```python
from build123d import *

# Parameters (mm, degrees)
SKETCH_W        = 19
SKETCH_H        = 14
PAD_DEPTH       = 19
THICKNESS_T     = 3
SKETCH001_R     = 1.5
POCKET_DEPTH    = 20
SKETCH002_R     = 1.5
POCKET001_DEPTH = 3
CHAMFER_SIZE    = 1.5
SKETCH003_W     = 19
SKETCH003_H     = 25
PAD001_DEPTH    = 1
POCKET002_DEPTH = 24


with BuildPart() as part:
    # Sketch → Pad (new body)
    with BuildSketch(Plane.XY):
        Rectangle(SKETCH_W, SKETCH_H)
    extrude(amount=PAD_DEPTH)

    # Thickness
    thickness_openings = [part.faces().sort_by_distance(p)[0] for p in [
        (-9.5, 0, 9.5),
        (9.5, 0, 9.5),
    ]]
    offset(amount=THICKNESS_T, openings=thickness_openings, kind=Kind.INTERSECTION)

    # Sketch001 (on Face8 of Thickness) → Pocket (cut)
    with BuildSketch(Plane.XZ.offset(10)):
        with Locations((0, 9.5)):
            Circle(SKETCH001_R)
    extrude(amount=-POCKET_DEPTH, mode=Mode.SUBTRACT)

    # Sketch002 (on Face10 of Pocket) → Pocket001 (cut)
    with BuildSketch(Plane.XZ.offset(10)):
        with Locations((-6.25, 9.5)):
            Circle(SKETCH002_R)
        with Locations((6.25, 9.5)):
            Circle(SKETCH002_R)
    extrude(amount=-POCKET001_DEPTH, mode=Mode.SUBTRACT)

    # Chamfer
    chamfer_edges = [part.edges().sort_by_distance(p)[0] for p in [
        (-9.5, 0, 0),
        (-9.5, 0, 19),
        (-9.5, 7, 9.5),
        (-9.5, -7, 9.5),
    ]]
    chamfer(chamfer_edges, length=CHAMFER_SIZE)

    # Sketch003 (on Face13 of Chamfer) → Pad001 (join)
    with BuildSketch(Plane(origin=(0, 10, 0), x_dir=(-1, 0, 0), z_dir=(0, 1, 0))):
        with Locations((0, 9.5)):
            Rectangle(SKETCH003_W, SKETCH003_H)
    extrude(amount=PAD001_DEPTH)

    # Sketch004 (on Face4 of Pad001) → Pocket002 (cut)
    with BuildSketch(Plane.YZ.offset(9.5)):
        with BuildLine():
            ThreePointArc((11, 19), (10.12132, 21.12132), (8, 22))
            Line((8, 22), (11, 22))
            Line((11, 22), (11, 19))
        make_face()
        with BuildLine():
            ThreePointArc((8, -3), (10.12132, -2.12132), (11, 0))
            Line((11, 0), (11, -3))
            Line((8, -3), (11, -3))
        make_face()
    extrude(amount=-POCKET002_DEPTH, mode=Mode.SUBTRACT)


solid = part.part
```
Geometry: final body of the model. Coordinates: model frame, mm. A direction names the side the tool comes from. Coordinates: 2 decimals unless noted, no trailing zeros. Write each loop counter-clockwise with the first axis right and the second up, starting at its lowest first coordinate (ties: lowest second). Pieces come first, ordered by that corner, then holes. Notation, with made-up numbers: M 84,-32 L 96,-32 A22 ccw 96,5 Z; hole C 53,-23 d2. An arc over 180 degrees is marked long. Answer as CSV lines item,"result". Start each with the question number.
Q1. Mould query, pull axis Y, two halves, no side actions, for faces 1 (the flat face through (1, 0, 0)), 2 (the flat face through (-2, -10, 9)), 3 (the cylindrical face through (5.06, -8.52, 8.59)). Classes: released by +Y, released by -Y, zero draft, split by the parting line, or undercut.
Q2. Line query: line 1 (Y direction, x = 5, z = 15.5); line 2 (Z direction, x = 0, y = -8.4); line 3 (Z direction, x = 6, y = 1.25). Output: solid intervals per line, ascending. Write a range as from..to.
Q3. Pin query (flat end, axial travel): P1, Ø2.5, axis at x = 0, z = 10, coming from the -Y side; P2, Ø2.5, axis at x = -6.25, z = 9.5, coming from the -Y side; P3, Ø12, axis at y = -0.5, z = 10.5, coming from the +X side (1 decimal). Return the tip coordinate at first contact, or that it passes through.
Q4. Cut plane D-D on y = -4.25. Return the cut outline in (x, z), then the cut area to 3 significant figures.
Q5. Cut plane A-A on z = 15.5. Return the cut outline in (x, y), then the cut area to 3 significant figures.
Q6. Cut plane C-C on z = 9.5. Return the cut outline in (x, y).
Q7. Cut plane B-B on x = 3. Return the cut outline in (y, z).
Q8. Reachability of faces 4 (the cylindrical face through (0, 8, 8)), 5 (the flat face through (-9, 0, -1)), 6 (the flat face through (1, 0, 19)) from +Z, -Z, +X, -X, +Y, -Y: full face, straight path, thin tool, end or side. Return the list, or none.
Findings below:
1,face 1,"undercut"
1,face 2,"released by -Y"
1,face 3,"zero draft"
2,line 1,"y = -10..-7, 7..11"
2,line 2,"z = -3..8, 11..22"
2,line 3,"z = -3..0, 19..22"
3,P1,"stops at y = -10"
3,P2,"stops at y = 7"
3,P3,"passes through"
4,outline,"M -9.5,-3 L 9.5,-3 L 9.5,0 L -8,0 L -9.5,-1.5 Z; M -9.5,20.5 L -8,19 L 9.5,19 L 9.5,22 L -9.5,22 Z"
4,area,"112 mm2"
5,outline,"M -9.5,-10 L 9.5,-10 L 9.5,-7 L -8,-7 L -9.5,-8.5 Z; M -9.5,8.5 L -8,7 L 9.5,7 L 9.5,11 L -9.5,11 Z"
5,area,"131 mm2"
6,outline,"M -9.5,-10 L -7.75,-10 L -7.75,-7 L -8,-7 L -9.5,-8.5 Z; M -9.5,8.5 L -8,7 L -1.5,7 L -1.5,10 L 1.5,10 L 1.5,7 L 9.5,7 L 9.5,11 L -9.5,11 Z; M -4.75,-10 L -1.5,-10 L -1.5,-7 L -4.75,-7 Z; M 1.5,-10 L 4.75,-10 L 4.75,-7 L 1.5,-7 Z; M 7.75,-10 L 9.5,-10 L 9.5,-7 L 7.75,-7 Z"
7,outline,"M -10,-3 L 8,-3 A3 ccw 11,0 L 11,19 A3 ccw 8,22 L -10,22 Z; hole M -7,0 L 7,0 L 7,19 L -7,19 Z"
8,face 4,"-Y"
8,face 5,"-X"
8,face 6,"+X, -X"
